Design review of the part built by this model. Coordinates are the model's own, in mm. A direction names the side the tool comes from. Give positions to 0.01 mm unless a question says otherwise; leave off trailing zeros. Write each loop counter-clockwise with the first axis right and the second up, starting at its lowest first coordinate (ties: lowest second). Pieces come first, ordered by that corner, then holes.
```python
from build123d import *


with BuildPart() as part:
    # Эскиз1 → Повернуть1 (revolve)
    with BuildSketch(Plane(origin=(0, 0, 0), x_dir=(1, 0, 0), z_dir=(0, 1, 0))):
        with BuildLine():
            Line((0, 0), (0, -33.35))
            ThreePointArc((0, -33.35), (-0.038268343, -33.342387953), (-0.070710678, -33.320710678))
            Line((-0.070710678, -33.320710678), (-0.75, -32.641421356))
            Line((-0.75, -32.641421356), (-0.75, -31.35))
            Line((-0.75, -31.35), (-0.495, -31.35))
            Line((-0.495, -31.35), (-0.495, -24.8))
            Line((-0.495, -24.8), (-0.68, -24.8))
            Line((-0.68, -24.8), (-0.68, -16.475))
            Line((-0.68, -16.475), (-0.579289322, -16.4))
            Line((-0.579289322, -16.4), (-0.68, -16.325))
            Line((-0.68, -16.325), (-0.68, -0.68))
            ThreePointArc((-0.68, -0.68), (-0.480832611, -0.199167389), (0, 0))
        make_face()
    revolve(axis=Axis((0, 0, 0), (0, 0, 1)))


solid = part.part
```
(1) Tool access review of faces 4 (the face through (-0.65, -0.2, 8.39)), 5 (the face through (0.75, -0.03, 31.99)): name each direction out of +Z, -Z, +X, -X, +Y, -Y from which nothing blocks a thin tool from reaching the whole face with its end or side.
Resolved:
face 4: -Z
face 5: +Z, -Z
(2) Consider section A-A, the plane z = 11.5. Give the boundary of the cut face in (x, y), then the cut area to 3 significant figures.
Resolved:
outline: circle Ø1.36 at (0, 0)
area: 1.45 mm2
(3) To check wall thickness, follow L1, parallel to Y at x = 0, z = 14.5; L2, parallel to Y at x = -0.2, z = 20. State the ranges of each line that lie inside material, in increasing order.
Resolved:
L1: y = -0.68 to 0.68
L2: y = -0.65 to 0.65
(4) Mouldability with a two-part tool opening along Z and no side actions: class faces 1 (the face through (-0.65, -0.2, 20.58)), 2 (the face through (0.041, 0.184, 33.203)), 3 (the face through (0.107, 0.483, 28.029)) as pulls with the +Z half, pulls with the -Z half, needs draft (parallel to the pull), parting line crosses it, or undercut.
Resolved:
face 1: needs draft
face 2: pulls with the +Z half
face 3: undercut
